Source: CAD feature listing. Evaluate the final solid. Frame: model axes, mm. Give positions to 0.01 mm unless a question says otherwise; leave off trailing zeros. Order: outer loops, then holes, each group sorted by start corner. A loop starts at its lowest first (then second) coordinate and runs counter-clockwise, first axis right, second up. Notation, with made-up numbers: M 78.5,38.25 L 98.5,38.25 A15 ccw 98.5,66.25 Z; hole C 70,-30.5 d3. An arc over 180 degrees is marked long. Use CSV: the item, a comma, the result in double quotes. Start each with the question number.
1. Section query D-D, the plane y = 92.75. Return the cut outline in (x, z), plus the area to 3 significant figures.
2. Line query: line 1 along X through (y, z) = (0.5, 1.9); line 2 along Y through (x, z) = (0, 2.2); line 3 along Y through (x, z) = (-2.5, 2.4). Output: solid intervals per line, ascending. Write a range as [from, to].
3. Pin query (flat end, axial travel): P1, Ø1.5, axis at x = 57, z = 1, coming from the -Y side; P2, Ø1.5, axis at x = -57, z = 1, coming from the -Y side; P3, Ø1, axis at x = 54, z = 2, coming from the +Y side. Return the tip coordinate at first contact, or that it passes through.
4. Mould query, pull axis Y, two halves, no side actions, for faces 1 (the cylindrical face through (-68.16, 73.17, 1.48)), 2 (the cylindrical face through (-59.641, 64.025, 1.479)), 3 (the flat face through (-60, 67, 0)). Classes: released by +Y, released by -Y, zero draft, split by the parting line, or undercut.
5. Section query A-A, the plane y = 0. Return the cut outline in (x, z), plus the area to 3 significant figures.
6. Section query C-C, the plane z = 2.55. Return the cut outline in (x, y), plus the area to 3 significant figures.
from build123d import *

# Parameters (mm, degrees)
SKETCH_1_R          = 100
SKETCH_1_R_2        = 87.5
SKETCH_1_R_3        = 3
EXTRUDE_1_DEPTH     = 3
CUT_EXTRUDE_1_DEPTH = 142.453172464


with BuildPart() as part:
    # 草图1 → 凸台-拉伸1 (new body)
    with BuildSketch(Plane.XY):
        Circle(SKETCH_1_R)
        Circle(SKETCH_1_R_2, mode=Mode.SUBTRACT)
        with Locations((0, 92.75)):
            Circle(SKETCH_1_R_3, mode=Mode.SUBTRACT)
        with Locations((92.75, 0)):
            Circle(SKETCH_1_R_3, mode=Mode.SUBTRACT)
        with Locations((0, -92.75)):
            Circle(SKETCH_1_R_3, mode=Mode.SUBTRACT)
        with Locations((-92.75, 0)):
            Circle(SKETCH_1_R_3, mode=Mode.SUBTRACT)
    extrude(amount=EXTRUDE_1_DEPTH)

    # 草图2 → 切除-拉伸1 (cut, through all)
    with BuildSketch(Plane.XY.offset(3)):
        with BuildLine():
            ThreePointArc((86.170678389, -15.194215546), (61.871843354, -61.871843354), (15.194215546, -86.170678389))
            Line((15.194215546, -86.170678389), (17.364817767, -98.480775301))
            ThreePointArc((17.364817767, -98.480775301), (70.710678119, -70.710678119), (98.480775301, -17.364817767))
            Line((98.480775301, -17.364817767), (86.170678389, -15.194215546))
        make_face()
    extrude(amount=-CUT_EXTRUDE_1_DEPTH, mode=Mode.SUBTRACT)


solid = part.part
Result set:
1,outline,"M -37.38,0 L -3,0 L -3,3 L -37.38,3 Z; M 3,0 L 37.38,0 L 37.38,3 L 3,3 Z"
1,area,"206 mm2"
2,line 1,"[-100, -95.71], [-89.79, -87.5], [87.5, 89.79], [95.71, 100]"
2,line 2,"[-100, -95.75], [-89.75, -87.5], [87.5, 89.75], [95.75, 100]"
2,line 3,"[-99.97, -94.41], [-91.09, -87.46], [87.46, 91.09], [94.41, 99.97]"
3,P1,"y = 65.74"
3,P2,"y = -82.68"
3,P3,"y = 84.49"
4,face 1,"split by the parting line"
4,face 2,"undercut"
4,face 3,"zero draft"
5,outline,"M -100,0 L -95.75,0 L -95.75,3 L -100,3 Z; M -89.75,0 L -87.5,0 L -87.5,3 L -89.75,3 Z; M 87.5,0 L 89.75,0 L 89.75,3 L 87.5,3 Z; M 95.75,0 L 100,0 L 100,3 L 95.75,3 Z"
5,area,"39.0 mm2"
6,outline,"M 15.19,-86.17 A87.5 cw long 86.17,-15.19 L 98.48,-17.36 A100 ccw long 17.36,-98.48 Z; hole C -92.75,0 d6; hole C 0,-92.75 d6; hole C 0,92.75 d6; hole C 92.75,0 d6"
6,area,"5,820 mm2"
